Source: CAD feature listing. Evaluate the final solid. Frame: model axes, mm. Face numbers are marked on the shaded views. A direction names the side the tool comes from. Round coordinates to 2 decimals unless told otherwise and drop trailing zeros. Order: outer loops, then holes, each group sorted by start corner. A loop starts at its lowest first (then second) coordinate and runs counter-clockwise, first axis right, second up. Notation, with made-up numbers: (71.5, 76) -> (113.5, 76) arc R15 ccw to (113.5, 99) -> close; hole circle Ø6 at (84.5, 49.5). An arc over 180 degrees is marked (long way). Answer as CSV lines item,"result".
from build123d import *

# Parameters (mm, degrees)
SKIZZE1_W                       = 300
SKIZZE1_H                       = 194.5
AUFSATZ_LINEAR_AUSTRAGEN1_DEPTH = 139
SKIZZE2_W                       = 290
SKIZZE2_H                       = 184.5
SCHNITT_LINEAR_AUSTRAGEN1_DEPTH = 134
F_8_0MM_STIFTLOCH1_D            = 8
SKIZZE8_W                       = 290
SKIZZE8_H                       = 184.5
SKIZZE8_W_2                     = 250
SKIZZE8_H_2                     = 144.5
AUFSATZ_LINEAR_AUSTRAGEN2_DEPTH = 25
AUFSATZ_LINEAR_AUSTRAGEN3_REACH = 211.377
SKIZZE9_W                       = 20
SKIZZE9_H                       = 20
SPIEGELN5_COPY_1_REACH          = 211.377
SPIEGELN5_COPY_1_SKETCH_W       = 20
SPIEGELN5_COPY_1_SKETCH_H       = 20
SKIZZE16_W                      = 290
SKIZZE16_H                      = 184.5
SKIZZE16_W_2                    = 250
SKIZZE16_H_2                    = 144.5
AUFSATZ_LINEAR_AUSTRAGEN4_DEPTH = 20


with BuildPart() as part:
    # Skizze1 → Aufsatz-Linear austragen1 (new body)
    with BuildSketch(Plane.XY):
        Rectangle(SKIZZE1_W, SKIZZE1_H)
    extrude(amount=AUFSATZ_LINEAR_AUSTRAGEN1_DEPTH)

    # Skizze2 → Schnitt-Linear austragen1 (cut)
    with BuildSketch(Plane(origin=(0, 0, 0), x_dir=(-1, 0, 0), z_dir=(0, 0, -1))):
        Rectangle(SKIZZE2_W, SKIZZE2_H)
    extrude(amount=-SCHNITT_LINEAR_AUSTRAGEN1_DEPTH, mode=Mode.SUBTRACT)

    # Ø8.0mm Stiftloch1 (through all)
    with Locations(Plane.ZY.offset(150)):
        with Locations((60, -42.25)):
            f_8_0mm_stiftloch1 = Hole(F_8_0MM_STIFTLOCH1_D / 2)

    # Spiegeln1: Ø8.0mm Stiftloch1 across plane
    add(f_8_0mm_stiftloch1.mirror(Plane.ZX), mode=Mode.SUBTRACT)

    # Skizze8 → Aufsatz-Linear austragen2 (add)
    with BuildSketch(Plane(origin=(0, 0, 30), x_dir=(-1, 0, 0), z_dir=(0, 0, -1))):
        Rectangle(SKIZZE8_W, SKIZZE8_H)
        Rectangle(SKIZZE8_W_2, SKIZZE8_H_2, mode=Mode.SUBTRACT)
    extrude(amount=AUFSATZ_LINEAR_AUSTRAGEN2_DEPTH)

    # Skizze9 → Aufsatz-Linear austragen3 (add, up to next)
    with BuildSketch(Plane(origin=(0, 0, 30), x_dir=(-1, 0, 0), z_dir=(0, 0, -1)), mode=Mode.PRIVATE) as aufsatz_linear_austragen3_sk1:
        with Locations((-135, -82.25)):
            Rectangle(SKIZZE9_W, SKIZZE9_H)
    aufsatz_linear_austragen3_tool1 = extrude(aufsatz_linear_austragen3_sk1.sketch, amount=-AUFSATZ_LINEAR_AUSTRAGEN3_REACH, mode=Mode.PRIVATE) - part.part
    aufsatz_linear_austragen3 = aufsatz_linear_austragen3_tool1.solids().sort_by_distance((135, -82.25, 30))[0]
    add(aufsatz_linear_austragen3)

    # Skizze15 → Kernloch für M4x0.71 (revolve, cut)
    with BuildSketch(Plane(origin=(135, -82.25, 5), x_dir=(0, 1, 0), z_dir=(1, 0, 0))):
        Polygon((0, 0), (0, 20.991420021), (1.65, 20), (1.65, 0), align=None)
    kernloch_f_r_m4x0_71 = revolve(axis=Axis((135, -82.25, -1.35), (0, 0, 1)), mode=Mode.SUBTRACT)

    # Spiegeln4: Aufsatz-Linear austragen3, Kernloch für M4x0.71 across plane
    add(aufsatz_linear_austragen3.mirror(Plane.ZX))
    add(kernloch_f_r_m4x0_71.mirror(Plane.ZX), mode=Mode.SUBTRACT)

    # Spiegeln5: Aufsatz-Linear austragen3, Kernloch für M4x0.71 across plane
    add(aufsatz_linear_austragen3.mirror(Plane(origin=(0, 0, 0), x_dir=(0, 0, 1), z_dir=(1, 0, 0))))
    add(kernloch_f_r_m4x0_71.mirror(Plane(origin=(0, 0, 0), x_dir=(0, 0, 1), z_dir=(1, 0, 0))), mode=Mode.SUBTRACT)

    # Spiegeln5 copy 1 sketch → Spiegeln5 copy 1 (add, up to next)
    with BuildSketch(Plane(origin=(0, 0, 30), x_dir=(1, 0, 0), z_dir=(0, 0, -1)), mode=Mode.PRIVATE) as spiegeln5_copy_1_sk1:
        with Locations((-135, -82.25)):
            Rectangle(SPIEGELN5_COPY_1_SKETCH_W, SPIEGELN5_COPY_1_SKETCH_H)
    spiegeln5_copy_1_tool1 = extrude(spiegeln5_copy_1_sk1.sketch, amount=-SPIEGELN5_COPY_1_REACH, mode=Mode.PRIVATE) - part.part
    add(spiegeln5_copy_1_tool1.solids().sort_by_distance((-135, 82.25, 30))[0])

    # Spiegeln5 copy 2 sketch → Spiegeln5 copy 2 (revolve, cut)
    with BuildSketch(Plane(origin=(-135, 82.25, 5), x_dir=(0, -1, 0), z_dir=(-1, 0, 0))):
        Polygon((0, 0), (0, 20.991420021), (1.65, 20), (1.65, 0), align=None)
    revolve(axis=Axis((-135, 82.25, -1.35), (0, 0, 1)), mode=Mode.SUBTRACT)

    # Skizze16 → Aufsatz-Linear austragen4 (add)
    with BuildSketch(Plane(origin=(0, 0, 134), x_dir=(-1, 0, 0), z_dir=(0, 0, -1))):
        Rectangle(SKIZZE16_W, SKIZZE16_H)
        Rectangle(SKIZZE16_W_2, SKIZZE16_H_2, mode=Mode.SUBTRACT)
    extrude(amount=AUFSATZ_LINEAR_AUSTRAGEN4_DEPTH)


solid = part.part
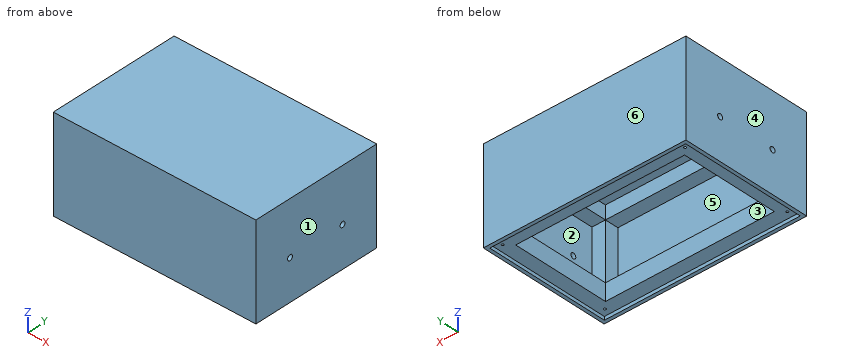
1. Reachability of the marked faces 1, 2 and 3 from +Z, -Z, +X, -X, +Y, -Y: full face, straight path, thin tool, end or side. Return the list, or none.
Results below:
face 1,"+Z, -Z, +X, +Y, -Y"
face 2,"none"
face 3,"-Z"
2. Section query B-B on y = -42.25. Return loops of the section in (x, z).
Results below:
outline,"(-150, 0) -> (-145, 0) -> (-145, 5) -> (-125, 5) -> (-125, 30) -> (-145, 30) -> (-145, 56) -> (-150, 56) -> close; (-150, 64) -> (-145, 64) -> (-145, 114) -> (-125, 114) -> (-125, 134) -> (125, 134) -> (125, 114) -> (145, 114) -> (145, 64) -> (150, 64) -> (150, 139) -> (-150, 139) -> close; (125, 5) -> (145, 5) -> (145, 0) -> (150, 0) -> (150, 56) -> (145, 56) -> (145, 30) -> (125, 30) -> close"
3. Pin query (flat end, axial travel): pin 1 (22 mm diameter, centred on x = 3, y = -78, fed in from -Z); pin 2 (7 mm diameter, centred on y = -42.25, z = 60, fed in from +X). Return the tip coordinate at first contact, or that it passes through.
Results below:
pin 1,"z = 5"
pin 2,"through"
4. Section query D-D on x = 50. Return loops of the section in (y, z).
Results below:
outline,"(-97.25, 0) -> (-92.25, 0) -> (-92.25, 5) -> (-72.25, 5) -> (-72.25, 30) -> (-92.25, 30) -> (-92.25, 114) -> (-72.25, 114) -> (-72.25, 134) -> (72.25, 134) -> (72.25, 114) -> (92.25, 114) -> (92.25, 30) -> (72.25, 30) -> (72.25, 5) -> (92.25, 5) -> (92.25, 0) -> (97.25, 0) -> (97.25, 139) -> (-97.25, 139) -> close"
5. Mould query, pull axis Y, two halves, no side actions, for the marked faces 4, 5 and 6. Classes: released by +Y, released by -Y, zero draft, split by the parting line, or undercut.
Results below:
face 4,"zero draft"
face 5,"undercut"
face 6,"released by +Y"
6. Section query C-C on z = 48.5. Return loops of the section in (x, y).
Results below:
outline,"(-150, -97.25) -> (150, -97.25) -> (150, 97.25) -> (-150, 97.25) -> close; hole (-145, -72.25) -> (-125, -72.25) -> (-125, -92.25) -> (125, -92.25) -> (125, -72.25) -> (145, -72.25) -> (145, 72.25) -> (125, 72.25) -> (125, 92.25) -> (-125, 92.25) -> (-125, 72.25) -> (-145, 72.25) -> close"
7. Line query: L1, parallel to X at y = -82, z = 9; L2, parallel to X at y = 13.5, z = 127.5; L3, parallel to Y at x = -135, z = 19.75. Output: solid intervals per line, ascending. Write a range as [from, to].
Results below:
L1,"[-150, -136.63], [-133.37, 133.37], [136.63, 150]"
L2,"[-150, -125], [125, 150]"
L3,"[-97.25, -83.9], [-80.6, 80.6], [83.9, 97.25]"
8. Section query A-A on z = 9. Return loops of the section in (x, y).
Results below:
outline,"(-150, -97.25) -> (150, -97.25) -> (150, 97.25) -> (-150, 97.25) -> close; hole circle Ø3.3 at (-135, -82.25); hole circle Ø3.3 at (-135, 82.25); hole (-125, -72.25) -> (125, -72.25) -> (125, 72.25) -> (-125, 72.25) -> close; hole circle Ø3.3 at (135, -82.25); hole circle Ø3.3 at (135, 82.25)"
